Here's the drawing with two shaded views (mm, measured from the low corner). I have some questions. A direction names the side the tool comes from. Coordinates: 2 decimals unless noted, no trailing zeros. Order: outer loops, then holes, each group sorted by start corner. A loop starts at its lowest first (then second) coordinate and runs counter-clockwise, first axis right, second up. Notation, with made-up numbers: (-5.75, 20.25) -> (33.25, 20.25) arc R12 ccw to (33.25, 40.25) -> close; hole circle Ø5 at (69.25, 89). An arc over 180 degrees is marked (long way). One line per item, written item: value. Start each with the question number.
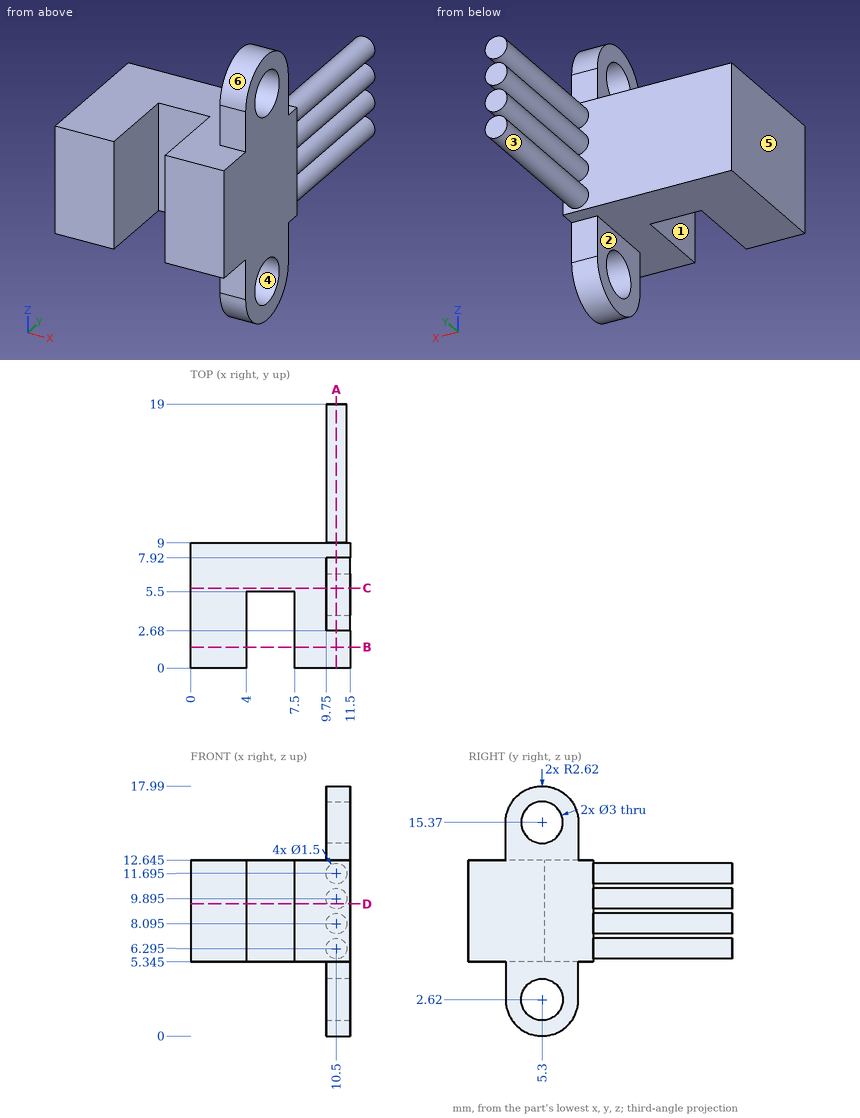
Q1. I need wall thicknesses on line 1 (Y direction, x = 10.7, z = 2.62); line 2 (X direction, y = 4.5, z = 11.25); line 3 (Z direction, x = 1, y = 7.25) (3 decimals). Which ranges of each line are inside material? Lowest first, please.
Q2. Imagine slicing it at B-B (y = 1.5). Write out the boundary of the cut face in (x, z) (3 decimals), plus the area to 3 significant figures.
Q3. Imagine slicing it at C-C (y = 5.75). Write out the boundary of the cut face in (x, z) (3 decimals), plus the area to 3 significant figures.
Q4. Imagine slicing it at D-D (z = 9.5). Write out the boundary of the cut face in (x, y).
Q5. Imagine slicing it at A-A (x = 10.5). Count the separate pieces of the cut face and the enclosed holes in it, plus the area to 3 significant figures.
Q6. For the marked faces 1, 2 and 3, which set-ups out of +Z, -Z, +X, -X, +Y, -Y let a thin tool reach every point of the face, with its end or its side?
Q7. If we mould it in two halves opening along Z, with no side actions, what happens to the marked faces 4, 5 and 6? For each: +Z half, -Z half, draft (parallel to the pull), parting line (faces both ways), or undercut.
Q8. For P1, Ø0.5, axis at x = 10.5, z = 4.5, coming from the -Y side; P2, Ø1.6, axis at y = 6.5, z = 14.5, coming from the -X side; P3, Ø3, axis at y = 16, z = 6, coming from the +X side, each with a flat end and sliding along its axis, tell me the tip position at first contact or that it passes through.
Completed:
1. line 1: y = 2.68 to 3.8, 6.8 to 7.92
1. line 2: x = 0 to 4, 7.5 to 11.5
1. line 3: z = 5.345 to 12.645
2. outline: (0, 5.345) -> (4, 5.345) -> (4, 12.645) -> (0, 12.645) -> close; (7.5, 5.345) -> (11.5, 5.345) -> (11.5, 12.645) -> (7.5, 12.645) -> close
2. area: 58.4 mm2
3. outline: (0, 5.345) -> (9.75, 5.345) -> (9.75, 4.051) -> (11.5, 4.051) -> (11.5, 13.939) -> (9.75, 13.939) -> (9.75, 12.645) -> (0, 12.645) -> close; (9.75, 0.039) -> (11.5, 0.039) -> (11.5, 1.189) -> (9.75, 1.189) -> close; (9.75, 16.801) -> (11.5, 16.801) -> (11.5, 17.951) -> (9.75, 17.951) -> close
3. area: 92.5 mm2
4. outline: (0, 0) -> (4, 0) -> (4, 5.5) -> (7.5, 5.5) -> (7.5, 0) -> (11.5, 0) -> (11.5, 9) -> (11.14, 9) -> (11.14, 19) -> (9.86, 19) -> (9.86, 9) -> (0, 9) -> close
5. separate pieces: 1
5. enclosed holes: 2
5. area: 162 mm2
6. face 1: +Z, -Z, -Y
6. face 2: -Z, -X, +Y, -Y
6. face 3: +Y
7. face 4: undercut
7. face 5: draft
7. face 6: +Z half
8. P1: stops at y = 2.68
8. P2: stops at x = 9.75
8. P3: stops at x = 11.25
